from build123d import *

# Parameters (mm, degrees)
REDONDEO3_R = 5


with BuildPart() as part:
    # Croquis1 → Revoluci_n1 (revolve)
    with BuildSketch(Plane(origin=(0, 0, 0), x_dir=(1, 0, 0), z_dir=(0, 1, 0)), mode=Mode.PRIVATE) as revoluci_n1_sk:
        with BuildLine():
            Line((106.445710743, 140), (70.03994637, 140))
            Line((70.03994637, 140), (48.737618848, 130.932753785))
            Line((48.737618848, 130.932753785), (48.737618848, 120.610275725))
            Line((48.737618848, 120.610275725), (31.868809424, 113.430137863))
            Line((31.868809424, 113.430137863), (31.868809424, 102.180137863))
            Line((31.868809424, 102.180137863), (15, 95))
            Line((15, 95), (15, 0))
            Line((15, 0), (70, 0))
            Line((70, 0), (126.445710743, 0))
            Line((126.445710743, 0), (126.445710743, 120))
            ThreePointArc((126.445710743, 120), (120.587846367, 134.142135624), (106.445710743, 140))
        make_face()
    revolve(revoluci_n1_sk.sketch.rotate(Axis((-209.218950064, 0, 0), (1, 0, 0)), 180), axis=Axis((-209.218950064, 0, 0), (1, 0, 0)))

    # Redondeo3
    redondeo3_edges = [part.edges().sort_by_distance(p)[0] for p in [
        (15, 0, -95),
        (31.868809424, 0, -102.180137863),
        (31.868809424, 0, -113.430137863),
        (48.737618848, 0, -120.610275725),
        (48.737618848, 0, -130.932753785),
    ]]
    fillet(redondeo3_edges, radius=REDONDEO3_R)


solid = part.part
Build history of the part. All positions in model axes, mm. A direction names the side the tool comes from. Round coordinates to 2 decimals unless told otherwise and drop trailing zeros. Write each loop counter-clockwise with the first axis right and the second up, starting at its lowest first coordinate (ties: lowest second). Pieces come first, ordered by that corner, then holes. Notation, with made-up numbers: (58.25, -3) - (115.25, -3) arc R30 ccw to (115.25, 19) - close; hole circle Ø8 at (74, -31.75). An arc over 180 degrees is marked (long way). One line per question, with ' | ' between items.
1. Band-saw the part on C-C, the plane x = 75. Write the cut outline in (y, z).
Results are:
outline: circle Ø280 at (0, 0)
2. Drop flat-ended pins along their axis: pin 1 Ø5 at (x, y) = (81.5, 40.5) entering from +Z; pin 2 Ø3 at (y, z) = (-107.5, 56.5) entering from -X; pin 3 Ø10 at (x, z) = (45.5, -105) entering from +Y. Give the stop position or say it passes through.
Results are:
pin 1: z = 134.74 | pin 2: x = 46.77 | pin 3: y = 81.17
3. Tool access for faces 1 (the face through (87.99, 136.67, -30.35)), 2 (the face through (31.869, 89, 57)): list every direction of +Z, -Z, +X, -X, +Y, -Y with a clear straight run to the whole face (end or side of a thin tool).
Results are:
face 1: +X, -X | face 2: -X
4. Drill centre lines: line 1 along X through (y, z) = (-93.5, -60); line 2 along Y through (x, z) = (104, -34); line 3 along Y through (x, z) = (64.5, 9). Where is each one in solid material? Low to high. Write a range as from..to.
Results are:
line 1: 31.96..126.45 | line 2: -135.81..135.81 | line 3: -137.35..137.35
5. Band-saw the part on A-A, the plane y = 0. Write the cut outline in (x, z).
Results are:
outline: (15, -91.69) arc R5 ccw to (18.04, -96.29) - (28.83, -100.89) arc R5 cw to (31.87, -105.49) - (31.87, -110.12) arc R5 ccw to (34.91, -114.72) - (45.7, -119.32) arc R5 cw to (48.74, -123.92) - (48.74, -127.63) arc R5 ccw to (51.78, -132.23) - (70.04, -140) - (106.45, -140) arc R20 ccw to (126.45, -120) - (126.45, 120) arc R20 ccw to (106.45, 140) - (70.04, 140) - (51.78, 132.23) arc R5 ccw to (48.74, 127.63) - (48.74, 123.92) arc R5 cw to (45.7, 119.32) - (34.91, 114.72) arc R5 ccw to (31.87, 110.12) - (31.87, 105.49) arc R5 cw to (28.83, 100.89) - (18.04, 96.29) arc R5 ccw to (15, 91.69) - close
